Part model, mm, in its own coordinate system. Face numbers are marked on the shaded views. Coordinates: 2 decimals unless noted, no trailing zeros. Write each loop counter-clockwise with the first axis right and the second up, starting at its lowest first coordinate (ties: lowest second). Pieces come first, ordered by that corner, then holes. Notation, with made-up numbers: (4, 83) -> (33, 83) arc R17 cw to (33, 99) -> close; hole circle Ø9 at (-33.5, 5). An arc over 180 degrees is marked (long way). Write item = value, one per line. Start each with the question number.
Q1. Pull direction Z, two halves, no side cores. Call the marked faces 1 and 2: released by +Z, released by -Z, zero draft, split by the parting line, or undercut.
Q2. Probe line 1 (X direction, y = 7.25, z = 0); line 2 (X direction, y = 0.15, z = 0); line 3 (Z direction, x = -20, y = 1). List the from-to ranges inside material, lowest first.
Q3. Band-saw the part on B-B, the plane x = 0. List the corners of the cut face in (y, z).
Q4. Band-saw the part on C-C, the plane y = 6. List the corners of the cut face in (x, z), plus the area to 3 significant figures.
Q5. Pin check, flat tips, straight feed: P1, Ø1.5, axis at y = 9, z = -15.5, coming from the -X side; P2, Ø1.5, axis at x = -11, y = 2.5, coming from the +Z side; P3, Ø2, axis at y = 8, z = 12, coming from the +X side. Stop position of each tip, or through.
Q6. Band-saw the part on A-A, the plane z = 0. List the corners of the cut face in (x, y).
from build123d import *

# Parameters (mm, degrees)
CROQUIS1_R              = 44
CROQUIS1_R_2            = 43.5
SALIENTE_EXTRUIR1_DEPTH = 12
CROQUIS2_R              = 44
CROQUIS2_R_2            = 42.8
SALIENTE_EXTRUIR2_DEPTH = 0.5
CHAFL_N1_SIZE           = 0.3


with BuildPart() as part:
    # Croquis1 → Saliente-Extruir1 (new body)
    with BuildSketch(Plane(origin=(0, 0, 0), x_dir=(1, 0, 0), z_dir=(0, 1, 0))):
        with Locations(Location((0, 0, 0), (0, 0, 270))):
            Circle(CROQUIS1_R)
        with Locations(Location((0, 0, 0), (0, 0, 270))):
            Circle(CROQUIS1_R_2, mode=Mode.SUBTRACT)
    extrude(amount=SALIENTE_EXTRUIR1_DEPTH)

    # Croquis2 → Saliente-Extruir2 (add)
    with BuildSketch(Plane.XZ):
        with Locations(Location((0, 0, 0), (0, 0, 90))):
            Circle(CROQUIS2_R)
        with Locations(Location((0, 0, 0), (0, 0, 270))):
            Circle(CROQUIS2_R_2, mode=Mode.SUBTRACT)
    extrude(amount=-SALIENTE_EXTRUIR2_DEPTH)

    # Chaflán1
    chafl_n1_edges = [part.edges().sort_by_distance(p)[0] for p in [
        (0, 0.5, 42.8),
        (0, 0.5, -43.5),
    ]]
    chamfer(chafl_n1_edges, length=CHAFL_N1_SIZE)


solid = part.part
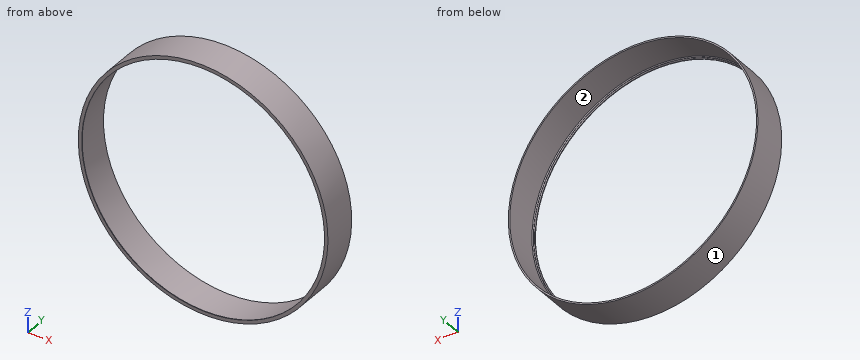
Ans:
q1.face_1 = split by the parting line
q1.face_2 = undercut
q2.line_1 = -44 to -43.5, 43.5 to 44
q2.line_2 = -44 to -42.8, 42.8 to 44
q2.line_3 = -39.19 to -38.63, 38.63 to 39.19
q3.outline = (0, -44) -> (12, -44) -> (12, -43.5) -> (0.8, -43.5) -> (0.5, -43.2) -> (0.5, -43.1) -> (0.2, -42.8) -> (0, -42.8) -> close; (0, 42.8) -> (0.2, 42.8) -> (0.5, 43.1) -> (0.5, 43.2) -> (0.8, 43.5) -> (12, 43.5) -> (12, 44) -> (0, 44) -> close
q4.outline = circle Ø88 at (0, 0); hole circle Ø87 at (0, 0)
q4.area = 137 mm2
q5.P1 = -41.45
q5.P2 = 42.79
q5.P3 = 42.6
q6.outline = (-44, 0) -> (-42.8, 0) -> (-42.8, 0.2) -> (-43.1, 0.5) -> (-43.2, 0.5) -> (-43.5, 0.8) -> (-43.5, 12) -> (-44, 12) -> close; (42.8, 0) -> (44, 0) -> (44, 12) -> (43.5, 12) -> (43.5, 0.8) -> (43.2, 0.5) -> (43.1, 0.5) -> (42.8, 0.2) -> close
